The model under review builds one solid part; all positions refer to its coordinate system, in mm. A direction names the side the tool comes from. Give positions to 0.01 mm unless a question says otherwise; leave off trailing zeros. Loops run counter-clockwise (first coordinate to the right, second up) from the corner with the lowest first, then second, coordinate; pieces in that order, holes last. Notation, with made-up numbers: M 6.5,72 L 12.5,72 A17 cw 12.5,89 Z; hole C 32,-2 d9. An arc over 180 degrees is marked long. Write item = value, one per line. Start each with the question number.
1. We need section B-B on y = 39. Give the boundary of the cut face in (x, z), then the cut area to 3 significant figures.
2. We need section C-C on x = 5. Give the boundary of the cut face in (y, z).
3. We need section A-A on z = 1.75. Count the separate pieces of the cut face and the enclosed holes in it, then the cut area to 3 significant figures.
4. For pin 1 (11 mm diameter, centred on x = 9, y = 62, fed in from -Z), flat-tipped, find the tip position at first contact; note if it passes through.
5. Wall thickness on line 1 along X through (y, z) = (-129.25, 3); line 2 along Y through (x, z) = (5, 2.5); line 3 along Y through (x, z) = (-14.5, 9): over which ranges is each line inside the solid? List them lowest first. Write a range as from..to.
6. For faces 1 (the face through (3.119, 4.725, 5.425)), 2 (the face through (5.432, 74.906, 3.451)), list the 3-axis set-ups (+Z, -Z, +X, -X, +Y, -Y) from which the entire face can be reached by the end or side of a thin tool; tool diameter is ignored.
from build123d import *

# Parameters (mm, degrees)
ESBO_O1_W                               = 90
ESBO_O1_H                               = 270
RESSALTO_EXTRUS_O1_DEPTH                = 10.7
FURO_ROSCADO_PARA_CONDU_TE_DE_M5X0_81_D = 5.2
FURO_ROSCADO_PARA_CONDU_TE_DE_1_4_281_D = 6.6294
FURO_ROSCADO_PARA_CONDU_TE_DE_M5X0_82_D = 5.2
FURO_ROSCADO_PARA_CONDU_TE_DE_10_321_D  = 5.1054
ESBO_O16_R                              = 11
CORTE_EXTRUS_O1_DEPTH                   = 7


with BuildPart() as part:
    # Esboço1 → Ressalto-extrusão1 (new body)
    with BuildSketch(Plane.XY):
        Rectangle(ESBO_O1_W, ESBO_O1_H)
    extrude(amount=RESSALTO_EXTRUS_O1_DEPTH)

    # Furo roscado para conduíte de M5x0.81 (through all)
    with Locations(Plane(origin=(0, 0, 0), x_dir=(-1, 0, 0), z_dir=(0, 0, -1))):
        with Locations((-40, -98.75), (-40, -129.25), (-14, -129.25), (-14, -98.75), (14, -98.75), (14, -129.25), (40, -129.25), (40, -98.75)):
            Hole(FURO_ROSCADO_PARA_CONDU_TE_DE_M5X0_81_D / 2)

    # Furo roscado para conduíte de 1/4-281 (through all)
    with Locations(Plane(origin=(0, 0, 0), x_dir=(-1, 0, 0), z_dir=(0, 0, -1))):
        with Locations((-20, -85), (20, -85)):
            Hole(FURO_ROSCADO_PARA_CONDU_TE_DE_1_4_281_D / 2)

    # Furo roscado para conduíte de M5x0.82 (through all)
    with Locations(Plane(origin=(0, 0, 0), x_dir=(-1, 0, 0), z_dir=(0, 0, -1))):
        with Locations((-35, 125), (-35, 20)):
            Hole(FURO_ROSCADO_PARA_CONDU_TE_DE_M5X0_82_D / 2)

    # Furo roscado para conduíte de #10-321 (through all)
    with Locations(Plane(origin=(0, 0, 0), x_dir=(-1, 0, 0), z_dir=(0, 0, -1))):
        with Locations((-5, 125), (-5, 89), (-5, 39), (-5, 3)):
            Hole(FURO_ROSCADO_PARA_CONDU_TE_DE_10_321_D / 2)

    # Esboço16 → Corte-extrusão1 (cut)
    with BuildSketch(Plane(origin=(0, 0, 0), x_dir=(-1, 0, 0), z_dir=(0, 0, -1))):
        with Locations((-4, 64)):
            Circle(ESBO_O16_R)
    extrude(amount=-CORTE_EXTRUS_O1_DEPTH, mode=Mode.SUBTRACT)


solid = part.part
Final values:
q1.outline = M -45,0 L 2.45,0 L 2.45,10.7 L -45,10.7 Z; M 7.55,0 L 45,0 L 45,10.7 L 7.55,10.7 Z
q1.area = 908 mm²
q2.outline = M -135,0 L 0.45,0 L 0.45,10.7 L -135,10.7 Z; M 5.55,0 L 36.45,0 L 36.45,10.7 L 5.55,10.7 Z; M 41.55,0 L 53.05,0 L 53.05,7 L 74.95,7 L 74.95,0 L 86.45,0 L 86.45,10.7 L 41.55,10.7 Z; M 91.55,0 L 122.45,0 L 122.45,10.7 L 91.55,10.7 Z; M 127.55,0 L 135,0 L 135,10.7 L 127.55,10.7 Z
q3.separate_pieces = 1
q3.enclosed_holes = 17
q3.area = 23,600 mm²
q4.pin_1 = 7
q5.line_1 = -45..-42.6, -37.4..-16.6, -11.4..11.4, 16.6..37.4, 42.6..45
q5.line_2 = -135..0.45, 5.55..36.45, 41.55..53.05, 74.95..86.45, 91.55..122.45, 127.55..135
q5.line_3 = -135..-131.8, -126.7..-101.3, -96.2..135
q6.face_1 = +Z, -Z
q6.face_2 = -Z
